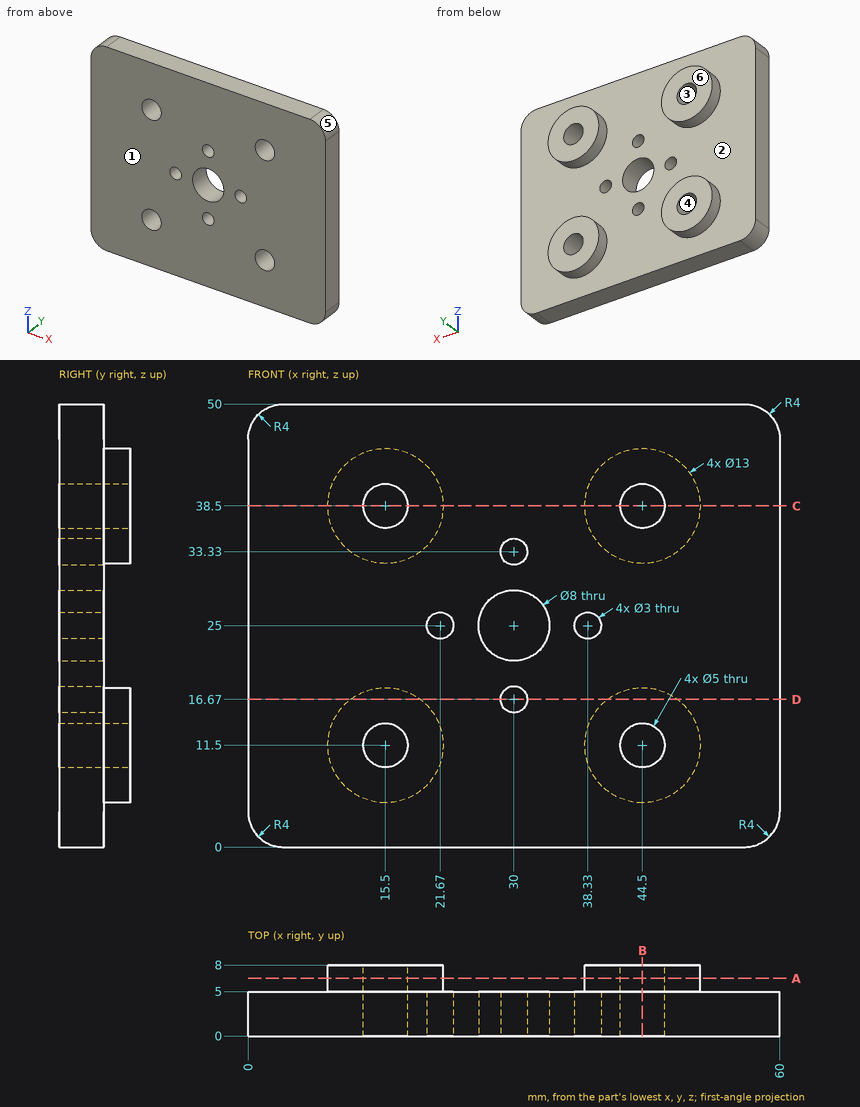
Design review of the part shown in the three views and the two pictorial views. Dimensions are in mm from the part's minimum x, y and z. A direction names the side the tool comes from. Give positions to 0.01 mm unless a question says otherwise; leave off trailing zeros. Loops run counter-clockwise (first coordinate to the right, second up) from the corner with the lowest first, then second, coordinate; pieces in that order, holes last. Notation, with made-up numbers: (69.25, 74.25) -> (74.25, 74.25) arc R17 cw to (74.25, 103.25) -> close; hole circle Ø1 at (-14.5, 6.5). An arc over 180 degrees is marked (long way). One line per item, written item: value.
Q1. We need section B-B on x = 44.5. Give the boundary of the cut face in (y, z), and give its area (3 significant figures).
Numbers:
outline: (0, 0) -> (5, 0) -> (5, 5) -> (8, 5) -> (8, 9) -> (0, 9) -> close; (0, 14) -> (8, 14) -> (8, 18) -> (5, 18) -> (5, 32) -> (8, 32) -> (8, 36) -> (0, 36) -> close; (0, 41) -> (8, 41) -> (8, 45) -> (5, 45) -> (5, 50) -> (0, 50) -> close
area: 248 mm^2
Q2. Draft analysis for pull direction Z (two halves, no side actions). For the marked faces 3, 4, 5 and 6, state which applies: pulls with the +Z half, pulls with the -Z half, needs draft (parallel to the pull), parting line crosses it, or undercut.
Numbers:
face 3: undercut
face 4: undercut
face 5: pulls with the +Z half
face 6: needs draft
Q3. We need section A-A on y = 6.5. Give the boundary of the cut face in (x, z), and give its area (3 significant figures).
Numbers:
outline: circle Ø13 at (15.5, 11.5); circle Ø13 at (15.5, 38.5); circle Ø13 at (44.5, 11.5); circle Ø13 at (44.5, 38.5); hole circle Ø5 at (15.5, 11.5); hole circle Ø5 at (15.5, 38.5); hole circle Ø5 at (44.5, 11.5); hole circle Ø5 at (44.5, 38.5)
area: 452 mm^2
Q4. For L1, parallel to X at y = 4.5, z = 11.5; L2, parallel to X at y = 3.1, z = 16.67; L3, parallel to Z at x = 17, y = 2, list the stretches that pass through material, from the lowest coordinate up.
Numbers:
L1: x = 0 to 13, 18 to 42, 47 to 60
L2: x = 0 to 28.5, 31.5 to 60
L3: z = 0 to 9.5, 13.5 to 36.5, 40.5 to 50
Q5. For pin 1 Ø3 at (x, z) = (44.5, 24) entering from +Y; pin 2 Ø4.5 at (x, z) = (15.5, 11.5) entering from -Y; pin 3 Ø1 at (x, y) = (11, 6) entering from -Z; pin 4 Ø1.5 at (y, z) = (7, 42) entering from +X, all flat-tipped, find the tip position at first contact; note any pin that passes through.
Numbers:
pin 1: stops at y = 5
pin 2: passes through
pin 3: stops at z = 6.38
pin 4: stops at x = 50.39
Q6. We need section C-C on z = 38.5. Give the boundary of the cut face in (x, y), and give its area (3 significant figures).
Numbers:
outline: (0, 0) -> (13, 0) -> (13, 8) -> (9, 8) -> (9, 5) -> (0, 5) -> close; (18, 0) -> (42, 0) -> (42, 8) -> (38, 8) -> (38, 5) -> (22, 5) -> (22, 8) -> (18, 8) -> close; (47, 0) -> (60, 0) -> (60, 5) -> (51, 5) -> (51, 8) -> (47, 8) -> close
area: 298 mm^2
Q7. Machinability: for the marked faces 1 and 2, which of the approach directions +Z, -Z, +X, -X, +Y, -Y give a long, thin tool a straight path to every point of the face, cutting with its end or side? Answer none if there is none.
Numbers:
face 1: +Z, -Z, +X, -X, -Y
face 2: +Y
Q8. We need section D-D on z = 16.67. Give the boundary of the cut face in (x, y), and give its area (3 significant figures).
Numbers:
outline: (0, 0) -> (28.5, 0) -> (28.5, 5) -> (19.44, 5) -> (19.44, 8) -> (11.56, 8) -> (11.56, 5) -> (0, 5) -> close; (31.5, 0) -> (60, 0) -> (60, 5) -> (48.44, 5) -> (48.44, 8) -> (40.56, 8) -> (40.56, 5) -> (31.5, 5) -> close
area: 332 mm^2
